Design review of the part built by this model. Coordinates are the model's own, in mm. A direction names the side the tool comes from. Give positions to 0.01 mm unless a question says otherwise; leave off trailing zeros. Order: outer loops, then holes, each group sorted by start corner. A loop starts at its lowest first (then second) coordinate and runs counter-clockwise, first axis right, second up. Notation, with made-up numbers: M -10,39 L 10,39 A27 cw 10,78 Z; hole C 87.25,74 d5. An arc over 180 degrees is marked long. Answer as a JSON object with one key per item and string values.
from build123d import *

# Parameters (mm, degrees)
SKETCH1_W           = 42
SKETCH1_H           = 99
SKETCH1_R           = 2
BOSS_EXTRUDE1_DEPTH = 8
CUT_EXTRUDE1_DEPTH  = 4
FILLET1_R           = 10


with BuildPart() as part:
    # Sketch1 → Boss-Extrude1 (new body)
    with BuildSketch(Plane(origin=(0, 0, 0), x_dir=(1, 0, 0), z_dir=(0, 1, 0))):
        with Locations((21, 49.5)):
            Rectangle(SKETCH1_W, SKETCH1_H)
        with Locations(Location((20, 77, 0), (0, 0, 270))):
            Circle(SKETCH1_R, mode=Mode.SUBTRACT)
        with Locations(Location((20, 22, 0), (0, 0, 270))):
            Circle(SKETCH1_R, mode=Mode.SUBTRACT)
    extrude(amount=BOSS_EXTRUDE1_DEPTH)

    # Sketch2 → Cut-Extrude1 (cut)
    with BuildSketch(Plane(origin=(0, 8, 0), x_dir=(1, 0, 0), z_dir=(0, 1, 0))):
        Polygon((21.876388375, 80.25), (18.123611625, 80.25), (16.24722325, 77), (18.123611625, 73.75), (21.876388375, 73.75), (23.75277675, 77), align=None)
        Polygon((21.876388375, 18.75), (23.75277675, 22), (21.876388375, 25.25), (18.123611625, 25.25), (16.24722325, 22), (18.123611625, 18.75), align=None)
    extrude(amount=-CUT_EXTRUDE1_DEPTH, mode=Mode.SUBTRACT)

    # Fillet1
    fillet1_edges = [part.edges().sort_by_distance(p)[0] for p in [
        (0, 4, 0),
        (0, 4, -99),
        (42, 4, -99),
        (42, 4, 0),
    ]]
    fillet(fillet1_edges, radius=FILLET1_R)


solid = part.part
(1) We need section B-B (x = 20). Write out the cut boundary in (y, z), plus the area to 3 significant figures.
Checked values:
{"outline": "M 0,-99 L 8,-99 L 8,-80.25 L 4,-80.25 L 4,-79 L 0,-79 Z; M 0,-75 L 4,-75 L 4,-73.75 L 8,-73.75 L 8,-25.25 L 4,-25.25 L 4,-24 L 0,-24 Z; M 0,-20 L 4,-20 L 4,-18.75 L 8,-18.75 L 8,0 L 0,0 Z", "area": "708 mm^2"}
(2) We need section D-D (x = 38). Write out the cut boundary in (y, z), plus the area to 3 significant figures.
Checked values:
{"outline": "M 0,-97 L 8,-97 L 8,-2 L 0,-2 Z", "area": "760 mm^2"}
(3) We need section C-C (y = 6.75). Write out the cut boundary in (x, z), plus the area to 3 significant figures.
Checked values:
{"outline": "M 0,-89 A10 ccw 10,-99 L 32,-99 A10 ccw 42,-89 L 42,-10 A10 ccw 32,0 L 10,0 A10 ccw 0,-10 Z; hole M 16.25,-77 L 18.12,-80.25 L 21.88,-80.25 L 23.75,-77 L 21.88,-73.75 L 18.12,-73.75 Z; hole M 16.25,-22 L 18.12,-25.25 L 21.88,-25.25 L 23.75,-22 L 21.88,-18.75 L 18.12,-18.75 Z", "area": "4,000 mm^2"}
(4) Draft analysis for pull direction X (two halves, no side actions). For faces 1 (the flat face through (20, 6, -80.25)), 2 (the flat face through (42, 4, -49)), 3 (the flat face through (0, 4, -49)), 4 (the flat face through (22, 4, -21)), state which applies: +X half, -X half, draft (parallel to the pull), parting line (faces both ways), or undercut.
Checked values:
{"face 1": "undercut", "face 2": "+X half", "face 3": "-X half", "face 4": "undercut"}
(5) We need section A-A (y = 2.5). Write out the cut boundary in (x, z), plus the area to 3 significant figures.
Checked values:
{"outline": "M 0,-89 A10 ccw 10,-99 L 32,-99 A10 ccw 42,-89 L 42,-10 A10 ccw 32,0 L 10,0 A10 ccw 0,-10 Z; hole C 20,-77 d4; hole C 20,-22 d4", "area": "4,050 mm^2"}
(6) Tool access review of faces 5 (the flat face through (20, 6, -73.75)), 6 (the cylindrical face through (20.601, 1.972, -75.092)): name each direction out of +Z, -Z, +X, -X, +Y, -Y from which nothing blocks a thin tool from reaching the whole face with its end or side.
Checked values:
{"face 5": "+Y", "face 6": "+Y, -Y"}
(7) To check wall thickness, follow L1, parallel to Z at x = 20, y = 0.9; L2, parallel to X at y = 3, z = -22; L3, parallel to Z at x = 19.5, y = 0.5. State the ranges of each line that lie inside material, in increasing order. Write a range as from..to.
Checked values:
{"L1": "z = -99..-79, -75..-24, -20..0", "L2": "x = 0..18, 22..42", "L3": "z = -99..-78.94, -75.06..-23.94, -20.06..0"}
